Input: dimensioned drawing with shaded views. Units: mm. Origin: part minimum x, y, z. A direction names the side the tool comes from. Round coordinates to 2 decimals unless told otherwise and drop trailing zeros. Order: outer loops, then holes, each group sorted by start corner. A loop starts at its lowest first (then second) coordinate and runs counter-clockwise, first axis right, second up.
Item 1: First-contact query: pin 1 (1.5 mm diameter, centred on x = 13.5, z = 8, fed in from +Y); pin 2 (6 mm diameter, centred on x = 59.5, y = 8.5, fed in from +Z); pin 3 (2 mm diameter, centred on x = 12.5, z = 3.5, fed in from -Y). Flat tips, straight axial feed; report the tip coordinate or a pass-through.
Item 2: Line query: L1, parallel to Y at x = 80.6, z = 12; L2, parallel to Y at x = 48.3, z = 0.35; L3, parallel to Z at x = 75.5, y = 24. Output: solid intervals per line, ascending.
Item 3: Reachability of the marked faces 1 and 2 from +Z, -Z, +X, -X, +Y, -Y: full face, straight path, thin tool, end or side. Return the list, or none.
Item 4: Cut plane B-B on z = 29.5. Output: boundary loops of the cut face in (x, y).
Item 5: Cut plane C-C on y = 15. Output: boundary loops of the cut face in (x, z).
Item 6: Cut plane D-D on x = 48.3. Output: boundary loops of the cut face in (y, z), then the cut area to 3 significant figures.
Item 7: Cut plane A-A on x = 16. Output: boundary loops of the cut face in (y, z).
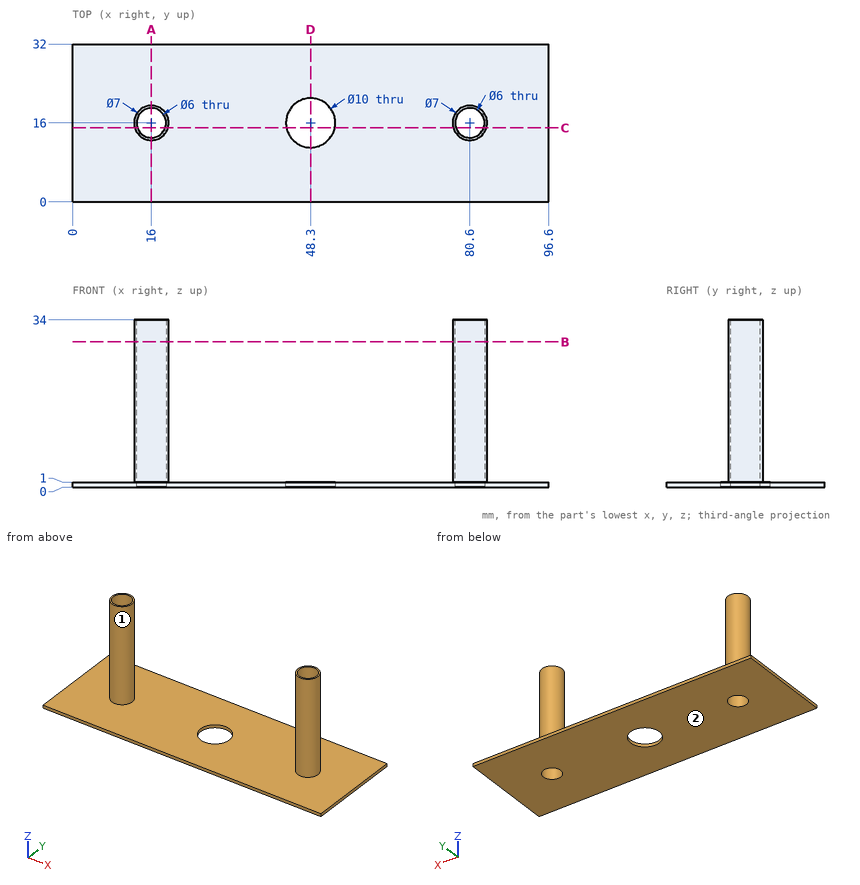
From the geometry:
1. pin 1: stops at y = 19.03
1. pin 2: stops at z = 1
1. pin 3: stops at y = 13.55
2. L1: y = 12.5 to 13, 19 to 19.5
2. L2: y = 0 to 11, 21 to 32
2. L3: z = 0 to 1
3. face 1: +Z
3. face 2: -Z, +X, -X, +Y, -Y
4. outline: circle Ø7 at (16, 16); circle Ø7 at (80.6, 16); hole circle Ø6 at (16, 16); hole circle Ø6 at (80.6, 16)
5. outline: (0, 0) - (13.17, 0) - (13.17, 34) - (12.65, 34) - (12.65, 1) - (0, 1) - close; (18.83, 0) - (43.4, 0) - (43.4, 1) - (19.35, 1) - (19.35, 34) - (18.83, 34) - close; (53.2, 0) - (77.77, 0) - (77.77, 34) - (77.25, 34) - (77.25, 1) - (53.2, 1) - close; (83.43, 0) - (96.6, 0) - (96.6, 1) - (83.95, 1) - (83.95, 34) - (83.43, 34) - close
6. outline: (0, 0) - (11, 0) - (11, 1) - (0, 1) - close; (21, 0) - (32, 0) - (32, 1) - (21, 1) - close
6. area: 22.0 mm2
7. outline: (0, 0) - (13, 0) - (13, 34) - (12.5, 34) - (12.5, 1) - (0, 1) - close; (19, 0) - (32, 0) - (32, 1) - (19.5, 1) - (19.5, 34) - (19, 34) - close
